```python
from build123d import *

# Parameters (mm, degrees)
F0_R     = 1.5875
F0_R_2   = 3.175
F1_DEPTH = 3.048


with BuildPart() as f1:
    # F0 (on Front) → F1 (new body)
    with BuildSketch(Plane.XZ):
        with BuildLine():
            Line((-9.450293, 115.490625), (-15.750488, 65.484375))
            ThreePointArc((-15.750488, 65.484375), (0, 79.375), (15.750488, 65.484375))
            Line((15.750488, 65.484375), (9.450293, 115.490625))
            ThreePointArc((9.450293, 115.490625), (9.506305, 114.896483), (9.525, 114.3))
            ThreePointArc((9.525, 114.3), (-0.596483, 104.793695), (-9.450293, 115.490625))
        make_face()
        with Locations((-5.664, 100.0252)):
            Circle(F0_R, mode=Mode.SUBTRACT)
        with BuildLine():
            ThreePointArc((-15.750488, 65.484375), (-15.863748, 64.097608), (-15.855144, 62.70625))
            ThreePointArc((-15.855144, 62.70625), (0, 47.625), (15.855144, 62.70625))
            ThreePointArc((15.855144, 62.70625), (15.870035, 63.103001), (15.875, 63.5))
            ThreePointArc((15.875, 63.5), (15.843841, 64.494139), (15.750488, 65.484375))
            ThreePointArc((15.750488, 65.484375), (0, 79.375), (-15.750488, 65.484375))
        make_face()
        with Locations((0, 63.5)):
            Circle(F0_R_2, mode=Mode.SUBTRACT)
        with BuildLine():
            ThreePointArc((-12.684115, -0.635), (-0.317599, 12.696028), (12.7, 0))
            ThreePointArc((12.7, 0), (9.449102, -8.485544), (1.360714, -12.626894))
            Line((1.360714, -12.626894), (45.300446, -7.891809))
            ThreePointArc((45.300446, -7.891809), (36.5125, 0), (45.300446, 7.891809))
            Line((45.300446, 7.891809), (20.747516, 10.537711))
            ThreePointArc((20.747516, 10.537711), (15.553195, 13.279782), (13.659067, 18.839656))
            Line((13.659067, 18.839656), (15.855144, 62.70625))
            ThreePointArc((15.855144, 62.70625), (0, 47.625), (-15.855144, 62.70625))
            Line((-15.855144, 62.70625), (-12.684115, -0.635))
        make_face()
        with BuildLine():
            ThreePointArc((1.360714, -12.626894), (9.449102, -8.485544), (12.7, 0))
            ThreePointArc((12.7, 0), (-0.317599, 12.696028), (-12.684115, -0.635))
            ThreePointArc((-12.684115, -0.635), (-8.246589, -9.658352), (1.360714, -12.626894))
        make_face()
        Circle(F0_R_2, mode=Mode.SUBTRACT)
        with BuildLine():
            ThreePointArc((45.300446, 7.891809), (36.5125, 0), (45.300446, -7.891809))
            ThreePointArc((45.300446, -7.891809), (50.355689, -5.303465), (52.3875, 0))
            ThreePointArc((52.3875, 0), (50.355689, 5.303465), (45.300446, 7.891809))
        make_face()
        with Locations((44.45, 0)):
            Circle(F0_R_2, mode=Mode.SUBTRACT)
        with BuildLine():
            ThreePointArc((9.450293, 115.490625), (0, 123.825), (-9.450293, 115.490625))
            ThreePointArc((-9.450293, 115.490625), (-0.596483, 104.793695), (9.525, 114.3))
            ThreePointArc((9.525, 114.3), (9.506305, 114.896483), (9.450293, 115.490625))
        make_face()
        with Locations((0, 114.3)):
            Circle(F0_R_2, mode=Mode.SUBTRACT)
    extrude(amount=F1_DEPTH)


solid = f1.part
```
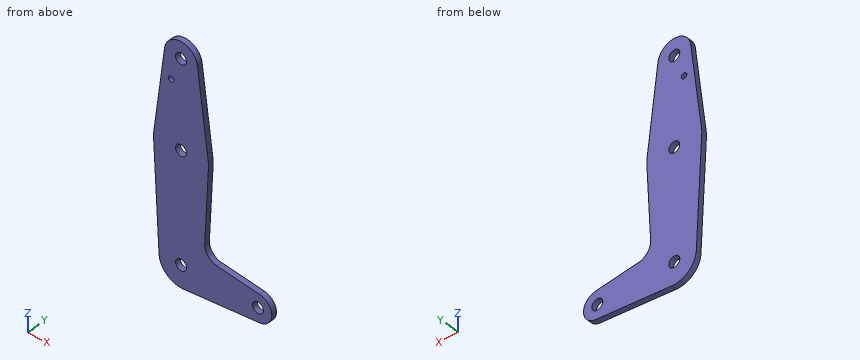
Here's how the part is built. I have some questions about the finished solid (model axes, mm). Coordinates: 2 decimals unless noted, no trailing zeros. Loops run counter-clockwise (first coordinate to the right, second up) from the corner with the lowest first, then second, coordinate; pieces in that order, holes last. Notation, with made-up numbers: (-29.75, -32) - (5.25, -32) arc R26 cw to (5.25, -7) - close; hole circle Ø4 at (-32, 14.5). An arc over 180 degrees is marked (long way). Answer as CSV lines item,"result".
Q1. If we section it at A-A, the plane x = 0: Write out the boundary of the cut face in (y, z) (3 decimals).
Response:
outline,"(-3.048, -12.7) - (0, -12.7) - (0, -3.175) - (-3.048, -3.175) - close; (-3.048, 3.175) - (0, 3.175) - (0, 60.325) - (-3.048, 60.325) - close; (-3.048, 66.675) - (0, 66.675) - (0, 111.125) - (-3.048, 111.125) - close; (-3.048, 117.475) - (0, 117.475) - (0, 123.825) - (-3.048, 123.825) - close"
Q2. If we section it at C-C, the plane z = 22.5: Write out the boundary of the cut face in (x, y), and give its area (3 significant figures).
Response:
outline,"(-13.84, -3.05) - (13.84, -3.05) - (13.84, 0) - (-13.84, 0) - close"
area,"84.4 mm2"
Q3. If we section it at B-B, the plane y = -1.3: Give the number of separate pieces and of enclosed holes in the cut face, and give its area (3 significant figures).
Response:
separate pieces,"1"
enclosed holes,"5"
area,"4,130 mm2"
Q4. If I drill on L1, parallel to Z at x = 0, y = -0.75 (3 decimals); L2, parallel to Z at x = -6.5, y = -0.15; L3, parallel to Z at x = -5, y = -0.85, over which ranges is the centre line in solid material (lowest first)? Write a range as [from, to].
Response:
L1,"[-12.7, -3.175], [3.175, 60.325], [66.675, 111.125], [117.475, 123.825]"
L2,"[-10.91, 98.68], [101.37, 121.26]"
L3,"[-11.67, 98.58], [101.47, 122.41]"
Q5. If we section it at D-D, the plane x = 34: Write out the boundary of the cut face in (y, z).
Response:
outline,"(-3.05, -9.11) - (0, -9.11) - (0, 9.11) - (-3.05, 9.11) - close"
Q6. For pin 1 (5 mm diameter, centred on x = 44.45, z = 0, fed in from -Y); pin 2 (1 mm diameter, centred on x = 11.5, y = -2.5, fed in from -Z); pin 3 (1.5 mm diameter, centred on y = -0.5, z = 102, fed in from -X), each with a flat end and sliding along its axis, tell me the tip position at first contact or that it passes through.
Response:
pin 1,"through"
pin 2,"z = -11.59"
pin 3,"x = -11.24"
